Source: CAD feature listing. Evaluate the final solid. Frame: model axes, mm. A direction names the side the tool comes from. Round coordinates to 2 decimals unless told otherwise and drop trailing zeros. Loops run counter-clockwise (first coordinate to the right, second up) from the corner with the lowest first, then second, coordinate; pieces in that order, holes last. Notation, with made-up numbers: M 72.25,-6.5 L 121.25,-6.5 A14 cw 121.25,11.5 Z; hole C 82.25,-36 d11. An arc over 180 degrees is marked long. Answer as a JSON object with one key per item and string values.
from build123d import *

# Parameters (mm, degrees)
ENL_V_MAT_EXTRU_1_DEPTH      = 12.9
ENL_V_MAT_EXTRU_1_DEPTH_BACK = 12.9
TROU_TARAUD_M4X0_71_D        = 3.3
TROU_TARAUD_M4X0_71_DEPTH    = 10
TROU_TARAUD_M4X0_71_TIP      = 0.991420021


with BuildPart() as part:
    # Esquisse1 → R_volution1 (revolve)
    with BuildSketch(Plane.XY, mode=Mode.PRIVATE) as r_volution1_sk:
        Polygon((0, -23), (21.5, -23), (24.5, -20), (24.5, 3), (22.5, 3), (22.5, 25.1), (22.2, 25.4), (0, 25.4), align=None)
    revolve(r_volution1_sk.sketch.rotate(Axis((0, 89.934503311, 0), (0, -1, 0)), 90), axis=Axis((0, 89.934503311, 0), (0, -1, 0)))

    # Esquisse2 → Enl_v. mat.-Extru.1 (cut, two sides: drawn at the far end of the back side and taken through both)
    with BuildSketch(Plane(origin=(0, 0, 0), x_dir=(0, 0, -1), z_dir=(1, 0, 0)).offset(-ENL_V_MAT_EXTRU_1_DEPTH_BACK)):
        Polygon((-24.5, -37), (24.5, 12), (24.5, 25.4), (-24.5, 25.4), align=None)
    extrude(amount=ENL_V_MAT_EXTRU_1_DEPTH + ENL_V_MAT_EXTRU_1_DEPTH_BACK, mode=Mode.SUBTRACT)

    # Trou taraud_ M4x0.71
    with Locations(Plane(origin=(0, 25.4, 0), x_dir=(-1, 0, 0), z_dir=(0, 1, 0))):
        with Locations((-19.5, 0), (19.5, 0)):
            Hole(TROU_TARAUD_M4X0_71_D / 2, depth=TROU_TARAUD_M4X0_71_DEPTH)
            with Locations((0, 0, -(TROU_TARAUD_M4X0_71_DEPTH + TROU_TARAUD_M4X0_71_TIP / 2))):  # 118° drill point
                Cone(0, TROU_TARAUD_M4X0_71_D / 2, TROU_TARAUD_M4X0_71_TIP, mode=Mode.SUBTRACT)


solid = part.part
Item 1: Section A-A on x = 0. Return the cut outline in (y, z), then the cut area to 3 significant figures.
Answer sheet:
{"outline": "M -23,-21.5 L -20,-24.5 L 3,-24.5 L 3,-22.5 L 10,-22.5 L -23,10.5 Z", "area": "592 mm²"}
Item 2: Line query: probe 1 along X at (y, z) = (17.75, 0); probe 2 along X at (y, z) = (-16, 6.5); probe 3 along X at (y, z) = (-6.5, 14.5). Output: solid intervals per line, ascending. Write a range as from..to.
Answer sheet:
{"probe 1": "x = -22.5..-21.15, -17.85..-12.9, 12.9..17.85, 21.15..22.5", "probe 2": "x = -23.62..-12.9, 12.9..23.62", "probe 3": "x = -19.75..-12.9, 12.9..19.75"}
Item 3: Access query for faces 1 (the flat face through (16, 25.4, 0)), 2 (the flat face through (5.3, 3, -22.1)), 3 (the flat face through (-0.2, -6.7, -5.8)). Directions: +Z, -Z, +X, -X, +Y, -Y. A direction counts if a zero-diameter tool reaches every point of the face in a straight line with its end or side. Return the directions, or none.
Answer sheet:
{"face 1": "+Z, -Z, +X, -X, +Y", "face 2": "+Y", "face 3": "+Z, +Y"}
Item 4: Contact query for flat-ended pins moving along their axis: pin 1 Ø3 at (y, z) = (17.5, 8) entering from -X; pin 2 Ø4 at (y, z) = (7, 13.5) entering from +X; pin 3 Ø1 at (x, y) = (-18, -17) entering from +Z. Output: stop coordinate, or through.
Answer sheet:
{"pin 1": "stops at x = -21.54", "pin 2": "stops at x = 19.34", "pin 3": "stops at z = 17.15"}
Item 5: Pull-direction query (Z, two-part tool) for faces 4 (the conical face through (-0.785, -22.812, -21.673)), 5 (the flat face through (-12.9, 7, 1)), 6 (the cylindrical face through (-20.81, 20.33, -1)), 7 (the conical face through (-19.8, 14.6, -0.1)); classes: pulls with the +Z half, pulls with the -Z half, needs draft (parallel to the pull), parting line crosses it, or undercut.
Answer sheet:
{"face 4": "parting line crosses it", "face 5": "needs draft", "face 6": "undercut", "face 7": "undercut"}
